Could you check a few things on this drawing? It's one solid part, dimensions in mm from its lowest x, y, z. Round coordinates to 2 decimals unless told otherwise and drop trailing zeros. Write each loop counter-clockwise with the first axis right and the second up, starting at its lowest first coordinate (ties: lowest second). Pieces come first, ordered by that corner, then holes. Notation, with made-up numbers: (-32, 88.25) - (-8, 88.25) arc R17 cw to (-8, 102.25) - close; hole circle Ø10 at (52.25, -20). An arc over 180 degrees is marked (long way). Use one line per item in the form item = value. Start each with the question number.
1. If I drill on line 1 along Z through (x, y) = (3.5, 14.75); line 2 along Z through (x, y) = (27.8, 13); line 3 along X through (y, z) = (14.5, 2), over which ranges is the centre line in solid material (lowest first)?
2. I want a section at A-A, the plane z = 5.5. List the corners of the cut face in (x, y) for me.
3. I want a section at C-C, the plane x = 3.5. List the corners of the cut face in (y, z) for me, plus the area to 3 significant figures.
4. Will these pins go through, and if not, where does the flat tip stop? pin 1 (10 mm diameter, centred on x = 40, y = 13, fed in from -Z); pin 2 (6 mm diameter, centred on y = 5, z = 2.5, fed in from +X); pin 3 (9 mm diameter, centred on x = 18.5, z = 6.5, fed in from -Y); pin 4 (5.5 mm diameter, centred on x = 27.8, z = 14.1, fed in from -Y).
5. I want a section at D-D, the plane y = 14. List the corners of the cut face in (x, z) for me.
6. I want a section at B-B, the plane x = 27.8. List the corners of the cut face in (y, z) for me.
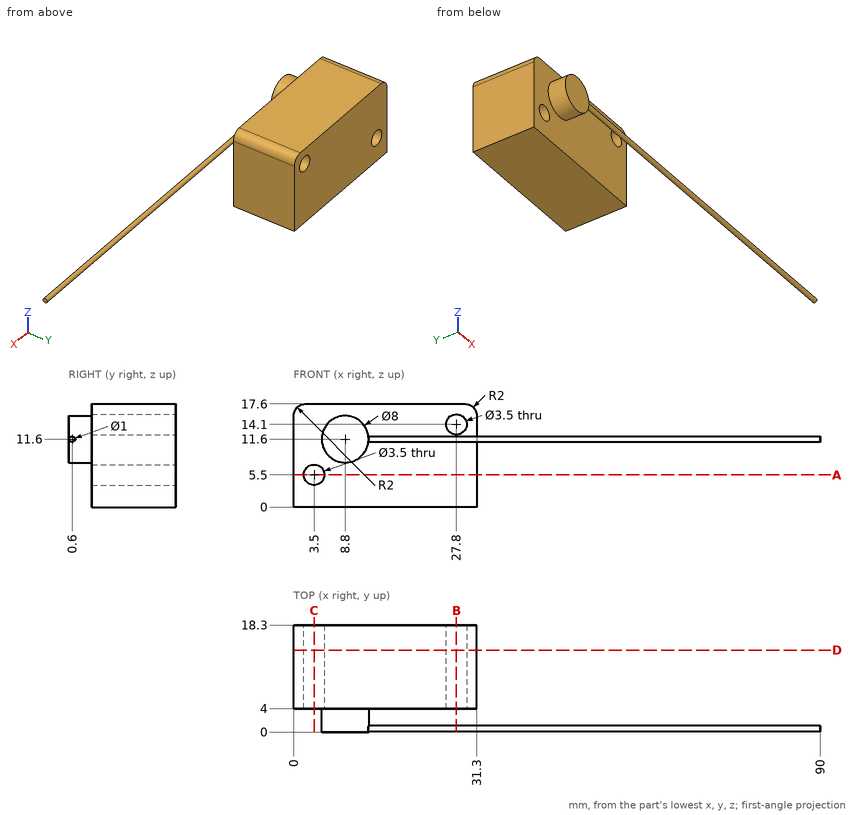
Model answer:
q1.line_1 = 0 to 3.75, 7.25 to 17.6
q1.line_2 = 0 to 12.35, 15.85 to 17.6
q1.line_3 = 0 to 31.3
q2.outline = (0, 4) - (1.75, 4) - (1.75, 18.3) - (0, 18.3) - close; (5.25, 4) - (31.3, 4) - (31.3, 18.3) - (5.25, 18.3) - close
q3.outline = (4, 0) - (18.3, 0) - (18.3, 3.75) - (4, 3.75) - close; (4, 7.25) - (18.3, 7.25) - (18.3, 17.6) - (4, 17.6) - close
q3.area = 202 mm2
q4.pin_1 = through
q4.pin_2 = 31.3
q4.pin_3 = 4
q4.pin_4 = 0.1
q5.outline = (0, 0) - (31.3, 0) - (31.3, 15.6) arc R2 ccw to (29.3, 17.6) - (2, 17.6) arc R2 ccw to (0, 15.6) - close; hole circle Ø3.5 at (3.5, 5.5); hole circle Ø3.5 at (27.8, 14.1)
q6.outline = circle Ø1 at (0.6, 11.6); (4, 0) - (18.3, 0) - (18.3, 12.35) - (4, 12.35) - close; (4, 15.85) - (18.3, 15.85) - (18.3, 17.6) - (4, 17.6) - close
